For this review, take the finished solid that the model builds, in its own axes (mm). Coordinates: 2 decimals unless noted, no trailing zeros. Loops run counter-clockwise (first coordinate to the right, second up) from the corner with the lowest first, then second, coordinate; pieces in that order, holes last. Notation, with made-up numbers: (52.5, 38) -> (77.5, 38) arc R24 cw to (77.5, 68) -> close; hole circle Ø2 at (46, 60.5). An arc over 180 degrees is marked (long way). Use a Markdown table: item, result.
from build123d import *

# Parameters (mm, degrees)
F0_W     = 59
F0_H     = 135.65
F1_DEPTH = 3.3
F2_R     = 1.5
F3_DEPTH = 3
F4_R     = 1.5
F5_DEPTH = 3


with BuildPart() as f1:
    # F0 (on Front) → F1 (new body)
    with BuildSketch(Plane.XZ):
        Rectangle(F0_W, F0_H)
    extrude(amount=F1_DEPTH)

    # F2 (on face) → F3 (cut)
    with BuildSketch(Plane(origin=(0, 0, 0), x_dir=(-1, 0, 0), z_dir=(0, 1, 0))):
        with Locations((14.5, 52.825)):
            Circle(F2_R)
        with Locations((14.5, -52.825)):
            Circle(F2_R)
    extrude(amount=-F3_DEPTH, mode=Mode.SUBTRACT)

    # F4 (on face) → F5 (cut)
    with BuildSketch(Plane(origin=(0, 0, 0), x_dir=(-1, 0, 0), z_dir=(0, 1, 0))):
        with Locations((-23.794, 27.362)):
            Circle(F4_R)
        with Locations((-11.021, 27.362)):
            Circle(F4_R)
        with Locations((-23.794, -39.138)):
            Circle(F4_R)
        with Locations((-11.021, -39.138)):
            Circle(F4_R)
    extrude(amount=-F5_DEPTH, mode=Mode.SUBTRACT)


solid = f1.part
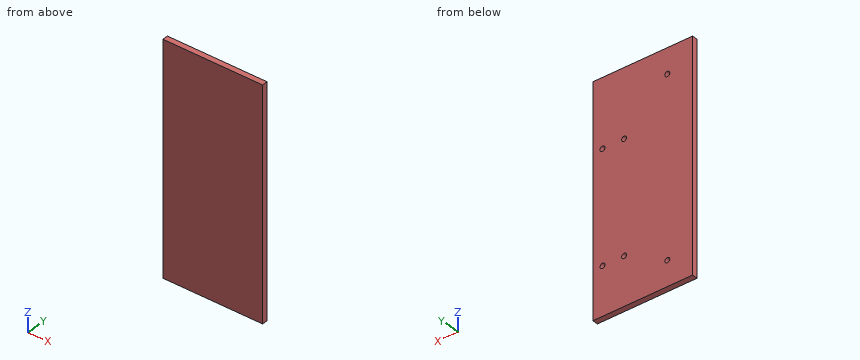
(1) For line 1 along Z through (x, y) = (-14.5, -1.15) (3 decimals); line 2 along Z through (x, y) = (23.5, -2.5) (3 decimals), list the stretches that pass through material, from the lowest coordinate up.
Found:
| item | result |
|---|---|
| line 1 | z = -67.825 to -54.325, -51.325 to 51.325, 54.325 to 67.825 |
| line 2 | z = -67.825 to -40.609, -37.667 to 25.891, 28.833 to 67.825 |
(2) Take a section at A-A on x = -14.5. Write out the cut boundary in (y, z) (3 decimals), plus the area to 3 significant figures.
Found:
| item | result |
|---|---|
| outline | (-3.3, -67.825) -> (0, -67.825) -> (0, -54.325) -> (-3, -54.325) -> (-3, -51.325) -> (0, -51.325) -> (0, 51.325) -> (-3, 51.325) -> (-3, 54.325) -> (0, 54.325) -> (0, 67.825) -> (-3.3, 67.825) -> close |
| area | 430 mm^2 |
(3) For pin 1 Ø2.5 at (x, z) = (-14.5, -52.825) entering from +Y, flat-tipped, find the tip position at first contact; note if it passes through.
Found:
| item | result |
|---|---|
| pin 1 | stops at y = -3 |
